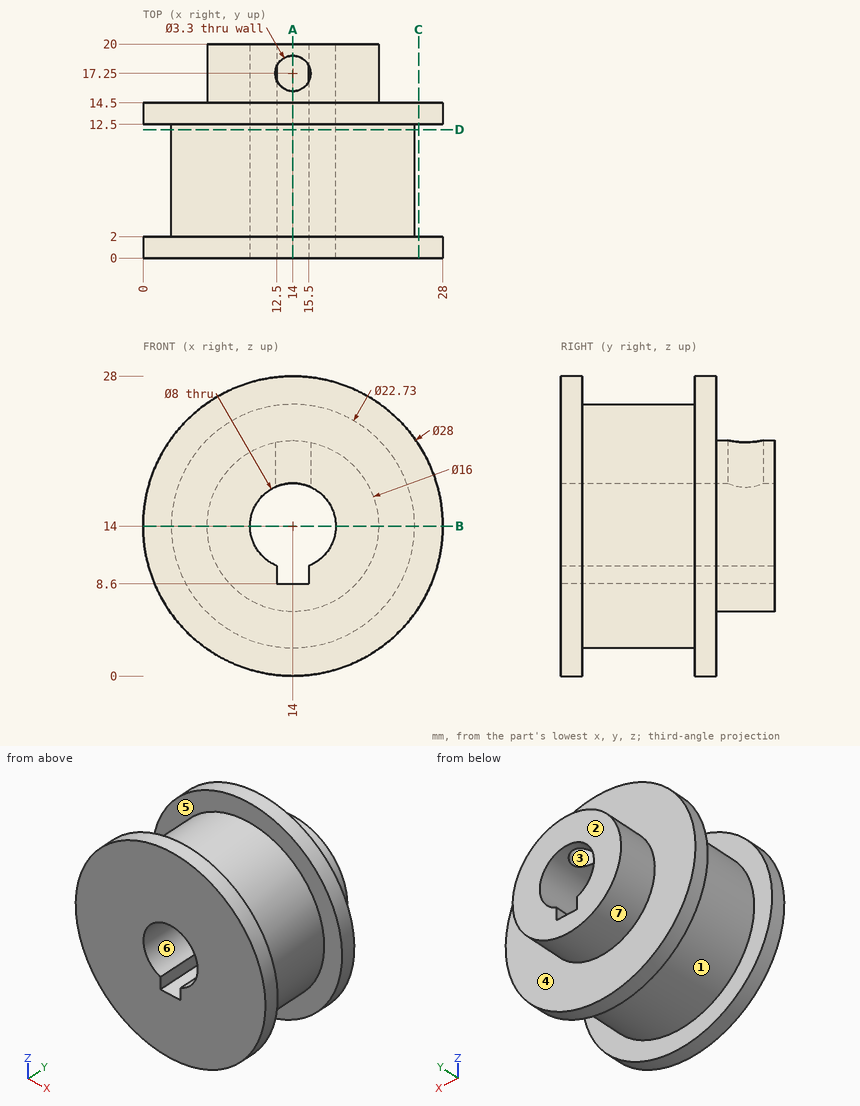
Check sheet for the drawn part. Datum: minimum x, y, z corner. Units: mm. A direction names the side the tool comes from. Round coordinates to 2 decimals unless told otherwise and drop trailing zeros. Order: outer loops, then holes, each group sorted by start corner. A loop starts at its lowest first (then second) coordinate and runs counter-clockwise, first axis right, second up.
1) Section check B-B (z = 14). Record the boundary of the cut face in (x, y) (3 decimals).
2) Tool access check on the marked faces 1, 2, 3 and 4. Record the directions out of +Z, -Z, +X, -X, +Y, -Y that give a thin tool (end or side, any length) a straight path to the whole face; none if there is none.
3) Section check C-C (x = 25.75). Record the boundary of the cut face in (y, z), and give its area (3 significant figures).
4) Scan lines: line 1 (Y direction, x = 2.5, z = 17.75); line 2 (Y direction, x = 14, z = 20.7); line 3 (X direction, y = 12.25, z = 14) (3 decimals). Record each from-to range of solid material in increasing order.
5) Mould release check, pull along X, two halves, no side actions. Record for the marked faces 5, 6 and 7: +X half, -X half, draft (parallel to the pull), parting line (faces both ways), or undercut.
6) Go/stop test with flat-tipped pins: pin 1 Ø5 at (x, y) = (19.5, 8) entering from +Z; pin 2 Ø4 at (x, y) = (15, 2.5) entering from -Z; pin 3 Ø3 at (x, y) = (14, 5) entering from -Z (3 decimals); pin 4 Ø2.5 at (x, y) = (14.5, 9.5) entering from +Z (3 decimals). Record where each tip stops, or that it passes through.
7) Section check A-A (x = 14). Record the boundary of the cut face in (y, z) (3 decimals).
8) Section check D-D (y = 12). Record the boundary of the cut face in (x, z) (3 decimals), and give its area (3 significant figures).
Result:
1. outline: (0, 0) - (10, 0) - (10, 20) - (6, 20) - (6, 14.5) - (0, 14.5) - (0, 12.5) - (2.635, 12.5) - (2.635, 2) - (0, 2) - close; (18, 0) - (28, 0) - (28, 2) - (25.365, 2) - (25.365, 12.5) - (28, 12.5) - (28, 14.5) - (22, 14.5) - (22, 20) - (18, 20) - close
2. face 1: none
2. face 2: +Z, -Z, +X, -X, +Y
2. face 3: +Z
2. face 4: +Y
3. outline: (0, 6.39) - (2, 6.39) - (2, 21.61) - (0, 21.61) - close; (12.5, 6.39) - (14.5, 6.39) - (14.5, 21.61) - (12.5, 21.61) - close
3. area: 60.9 mm2
4. line 1: y = 0 to 2, 12.5 to 14.5
4. line 2: y = 0 to 15.6, 18.9 to 20
4. line 3: x = 2.635 to 10, 18 to 25.365
5. face 5: draft
5. face 6: undercut
5. face 7: parting line
6. pin 1: stops at z = 24.96
6. pin 2: stops at z = 0
6. pin 3: stops at z = 2.635
6. pin 4: stops at z = 25.365
7. outline: (0, 0) - (2, 0) - (2, 2.635) - (12.5, 2.635) - (12.5, 0) - (14.5, 0) - (14.5, 6) - (20, 6) - (20, 8.6) - (0, 8.6) - close; (0, 18) - (15.6, 18) - (15.6, 22) - (14.5, 22) - (14.5, 28) - (12.5, 28) - (12.5, 25.365) - (2, 25.365) - (2, 28) - (0, 28) - close; (18.9, 18) - (20, 18) - (20, 22) - (18.9, 22) - close
8. outline: circle Ø22.73 at (14, 14); hole (12.5, 8.6) - (15.5, 8.6) - (15.5, 10.292) arc R4 ccw (long way) to (12.5, 10.292) - close
8. area: 351 mm2
